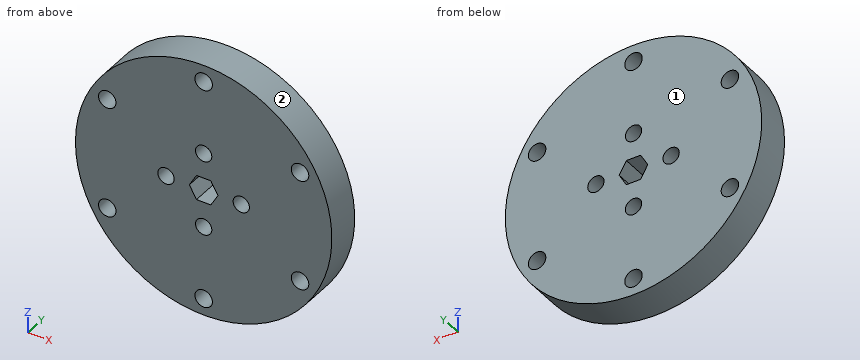
Autodesk Inventor part; units mm, degrees
ref_plane "YZ Plane" through (0, 0, 0) normal (1, 0, 0) x (0, 1, 0)
ref_plane "XZ Plane" through (0, 0, 0) normal (0, 1, 0) x (-1, 0, 0)
ref_plane "XY Plane" through (0, 0, 0) normal (0, 0, 1) x (1, 0, 0)
sketch "Sketch1" plane through (0, 0, 0) normal (0, 1, 0) x (-1, 0, 0)
  circle A0 centre (0, 0) radius 27.94
  dimension "d0" = 55.88
extrude "Extrusion1" add sketch "Sketch1" along normal blind 7.62
ref_plane "Work Plane5" through (0, 21.082, 0) normal (0, 1, 0) x (1, 0, 0)
sketch "Sketch5" plane through (0, 21.082, 0) normal (0, 1, 0) x (1, 0, 0)
  line L0 (0, 0) -> (0, 2.667)
  line L1 (-3.1168, 0) -> (-1.5584, 2.6992)
  line L2 (-1.5584, 2.6992) -> (1.5584, 2.6992)
  line L3 (1.5584, 2.6992) -> (3.1168, 0)
  line L4 (3.1168, 0) -> (1.5584, -2.6992)
  line L5 (1.5584, -2.6992) -> (-1.5584, -2.6992)
  line L6 (-1.5584, -2.6992) -> (-3.1168, 0)
  dimension "d10" = 2.667
extrude "Extrusion4" cut sketch "Sketch5" against normal blind 25.4
sketch "Sketch6" plane through (0, 7.62, 0) normal (0, 1, 0) x (1, 0, 0)
  circle A0 centre (0, 0) radius 27.94
  line L0 (0, -27.94) -> (0, -26.162)
  line L1 (0, -26.162) -> (0, -24.257)
  circle A1 centre (0, -24.257) radius 1.905
  dimension "d13" = 1.778
  dimension "d14" = 1.905
extrude "Extrusion5" cut sketch "Sketch6" against normal blind 25.4 contours A1
ref_plane "Work Plane6" through (0, 21.082, 0) normal (0, 1, 0) x (1, 0, 0)
pattern_circular "Circular Pattern1" count 6 over 360 about axis through (0, 21.082, 0) along (0, 1, 0) of "Extrusion5"
sketch "Sketch8" plane through (0, 0, 0) normal (0, -1, 0) x (1, 0, 0)
  line L0 (3.1168, 0) -> (1.5584, -2.6992)
  line L1 (3.1168, 0) -> (6.4188, 0)
  line L2 (6.4188, 0) -> (8.1968, 0)
  circle A0 centre (8.1968, 0) radius 1.778
  point P0 (0, 0)
  dimension "d20" = 3.302
  dimension "d21" = 1.778
extrude "Extrusion6" cut sketch "Sketch8" against normal blind 25.4
pattern_circular "Circular Pattern2" count 4 over 360 about axis through (0, 21.082, 0) along (0, 1, 0) of "Extrusion6"
properties part number "Wheel Mount"
Check sheet for the modelled part. Datum: model origin and axes. Units: mm. Face numbers are marked on the shaded views. Coordinates: 2 decimals unless noted, no trailing zeros. Order: outer loops, then holes, each group sorted by start corner. A loop starts at its lowest first (then second) coordinate and runs counter-clockwise, first axis right, second up. Notation, with made-up numbers: (13.25, 27) -> (26.25, 27) arc R25 cw to (26.25, 39) -> close; hole circle Ø1 at (80, -4). An arc over 180 degrees is marked (long way). Write each question's results on one line, items separated by ' | '. Start each with the question number.
1) Material ranges on line 1 along Z through (x, y) = (0, 5.75); line 2 along X through (y, z) = (7, -12.5); line 3 along Z through (x, y) = (21.5, 6), recorded low to high.
2) Section check D-D (z = -17). Enter the section's corners in (x, y).
3) Section check B-B (x = -8). Enter the section's corners in (y, z), and give its area (3 significant figures).
4) Section check A-A (x = 0). Enter the section's corners in (y, z), and give its area (3 significant figures).
5) Depth check by flat-ended pin: pin 1 (2.5 mm diameter, centred on x = 21.01, z = 12.13, fed in from +Y); pin 2 (2 mm diameter, centred on y = 5.5, z = -12, fed in from +X); pin 3 (1.6 mm diameter, centred on x = 0, y = 3, fed in from +Z); pin 4 (1.5 mm diameter, centred on y = 4, z = -15.5, fed in from +X). Enter the tip coordinate at first touch or a pass-through.
6) Section check C-C (y = 6.75). Count the separate pieces of the cut face and the enclosed holes in it, and give its area (3 significant figures).
7) Draft check along X on the marked faces 1 and 2. Enter one of: pulls with the +X half, pulls with the -X half, needs draft (parallel to the pull), parting line crosses it, or undercut.
Checked values:
1) line 1: -27.94 to -26.16, -22.35 to -9.97, -6.42 to -2.7, 2.7 to 6.42, 9.97 to 22.35, 26.16 to 27.94 | line 2: -24.99 to -22.88, -19.14 to 19.14, 22.88 to 24.99 | line 3: -17.84 to -13.97, -10.29 to 10.29, 13.97 to 17.84
2) outline: (-22.17, 0) -> (22.17, 0) -> (22.17, 7.62) -> (-22.17, 7.62) -> close
3) outline: (0, -26.77) -> (7.62, -26.77) -> (7.62, -1.77) -> (0, -1.77) -> close; (0, 1.77) -> (7.62, 1.77) -> (7.62, 26.77) -> (0, 26.77) -> close | area: 381 mm²
4) outline: (0, -27.94) -> (7.62, -27.94) -> (7.62, -26.16) -> (0, -26.16) -> close; (0, -22.35) -> (7.62, -22.35) -> (7.62, -9.97) -> (0, -9.97) -> close; (0, -6.42) -> (7.62, -6.42) -> (7.62, -2.7) -> (0, -2.7) -> close; (0, 2.7) -> (7.62, 2.7) -> (7.62, 6.42) -> (0, 6.42) -> close; (0, 9.97) -> (7.62, 9.97) -> (7.62, 22.35) -> (0, 22.35) -> close; (0, 26.16) -> (7.62, 26.16) -> (7.62, 27.94) -> (0, 27.94) -> close | area: 272 mm²
5) pin 1: through | pin 2: x = 25.68 | pin 3: z = 27.94 | pin 4: x = 23.73
6) separate pieces: 1 | enclosed holes: 11 | area: 2,320 mm²
7) face 1: needs draft | face 2: parting line crosses it
